CAD build for the part. Positions are in the model's coordinates, mm. Face numbers are marked on the shaded views. A direction names the side the tool comes from. Coordinates: 2 decimals unless noted, no trailing zeros. Loops run counter-clockwise (first coordinate to the right, second up) from the corner with the lowest first, then second, coordinate; pieces in that order, holes last. Notation, with made-up numbers: (-15.5, -27) - (15.5, -27) arc R7 ccw to (15.5, -15) - close; hole circle Ø5 at (3.25, 53.5). An arc over 180 degrees is marked (long way). Put each result on its own line as item: value.
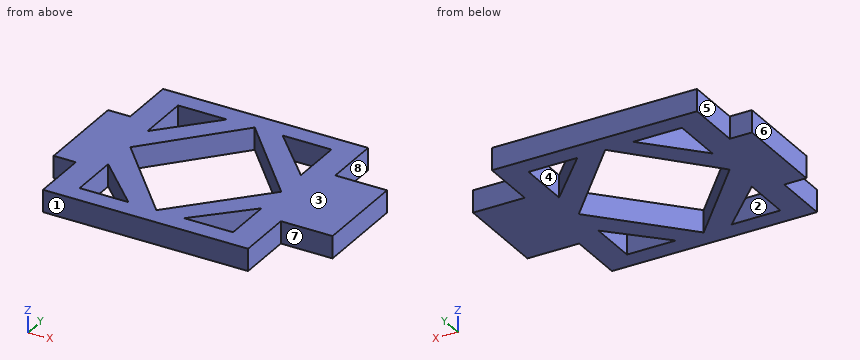
```python
from build123d import *

# Parameters (mm, degrees)
SALIENTE_EXTRUIR1_DEPTH = 3


with BuildPart() as part:
    # Croquis1 → Saliente-Extruir1 (new body)
    with BuildSketch(Plane.XY):
        Polygon((97.334837859, 52.056418279), (97.334837859, 39.456418279), (100.334837859, 39.456418279), (100.334837859, 31.871418279), (128.104837859, 31.871418279), (128.104837859, 39.456418279), (135.104837859, 39.456418279), (135.104837859, 52.056418279), (128.104837859, 52.056418279), (128.104837859, 59.641418279), (100.334837859, 59.641418279), (100.334837859, 52.056418279), align=None)
        Polygon((110.434837859, 57.141418279), (103.834837859, 57.141418279), (103.834837859, 50.071418279), align=None, mode=Mode.SUBTRACT)
        Polygon((103.834837859, 40.971418279), (103.834837859, 34.371418279), (110.434837859, 34.371418279), align=None, mode=Mode.SUBTRACT)
        Polygon((118.004837859, 34.371418279), (124.604837859, 34.371418279), (124.604837859, 40.971418279), align=None, mode=Mode.SUBTRACT)
        Polygon((124.604837859, 50.076418279), (124.604837859, 57.141418279), (118.004837859, 57.141418279), align=None, mode=Mode.SUBTRACT)
        Polygon((114.219837859, 57.141418279), (124.604837859, 45.523918279), (114.219837859, 34.371418279), (104.042671946, 45.756418279), align=None, mode=Mode.SUBTRACT)
    extrude(amount=SALIENTE_EXTRUIR1_DEPTH)


solid = part.part
```
Q1. Slice it at D-D, the plane x = 112. Give the cut face in (y, z), then the cut area to 3 significant figures.
Determined:
outline: (31.87, 0) - (36.85, 0) - (36.85, 3) - (31.87, 3) - close; (54.66, 0) - (59.64, 0) - (59.64, 3) - (54.66, 3) - close
area: 29.9 mm2
Q2. Tool access for the marked faces 4, 5, 6, 7 and 8: list every direction of +Z, -Z, +X, -X, +Y, -Y with a clear straight run to the whole face (end or side of a thin tool).
Determined:
face 4: +Z, -Z
face 5: +Z, -Z, -X, +Y
face 6: +Z, -Z, -X, +Y, -Y
face 7: +Z, -Z, +X, -Y
face 8: +Z, -Z, +X, +Y
Q3. Pin check, flat tips, straight feed: pin 1 Ø1.5 at (y, z) = (53.5, 2) entering from +X; pin 2 Ø1.5 at (x, z) = (98.5, 1.5) entering from +Y; pin 3 Ø0.9 at (x, z) = (99, 1) entering from -Y. Stop position of each tip, or through.
Determined:
pin 1: x = 128.1
pin 2: y = 52.06
pin 3: y = 39.46
Q4. Slice it at C-C, the plane z = 0.7. Give the cut face in (x, y), then the cut area to 3 significant figures.
Determined:
outline: (97.33, 39.46) - (100.33, 39.46) - (100.33, 31.87) - (128.1, 31.87) - (128.1, 39.46) - (135.1, 39.46) - (135.1, 52.06) - (128.1, 52.06) - (128.1, 59.64) - (100.33, 59.64) - (100.33, 52.06) - (97.33, 52.06) - close; hole (103.83, 34.37) - (110.43, 34.37) - (103.83, 40.97) - close; hole (103.83, 50.07) - (110.43, 57.14) - (103.83, 57.14) - close; hole (104.04, 45.76) - (114.22, 34.37) - (124.6, 45.52) - (114.22, 57.14) - close; hole (118, 34.37) - (124.6, 34.37) - (124.6, 40.97) - close; hole (118, 57.14) - (124.6, 50.08) - (124.6, 57.14) - close
area: 573 mm2
Q5. Mould opens along Y. For the marked faces 1, 2 and 3 say: +Y half, -Y half, draft (parallel to the pull), parting line (faces both ways), or undercut.
Determined:
face 1: -Y half
face 2: undercut
face 3: draft
Q6. Wall check: L1, parallel to X at y = 51, z = 2.7; L2, parallel to Y at x = 106.5, z = 2.55; L3, parallel to Y at x = 121.5, z = 1.9. Give the ranges that are in metal, low to high. Write a range as from..to.
Determined:
L1: 97.33..103.83, 104.7..108.73, 119.71..123.74, 124.6..135.1
L2: 31.87..34.37, 38.31..43.01, 48.51..52.93, 57.14..59.64
L3: 31.87..34.37, 37.87..42.19, 49..53.4, 57.14..59.64
Q7. Slice it at A-A, the plane x = 120. Give the cut face in (y, z), then the cut area to 3 significant figures.
Determined:
outline: (31.87, 0) - (34.37, 0) - (34.37, 3) - (31.87, 3) - close; (36.37, 0) - (40.58, 0) - (40.58, 3) - (36.37, 3) - close; (50.68, 0) - (55.01, 0) - (55.01, 3) - (50.68, 3) - close; (57.14, 0) - (59.64, 0) - (59.64, 3) - (57.14, 3) - close
area: 40.6 mm2
Q8. Slice it at B-B, the plane y = 55. Give the cut face in (x, z).
Determined:
outline: (100.33, 0) - (103.83, 0) - (103.83, 3) - (100.33, 3) - close; (108.44, 0) - (112.31, 0) - (112.31, 3) - (108.44, 3) - close; (116.13, 0) - (120.01, 0) - (120.01, 3) - (116.13, 3) - close; (124.6, 0) - (128.1, 0) - (128.1, 3) - (124.6, 3) - close
